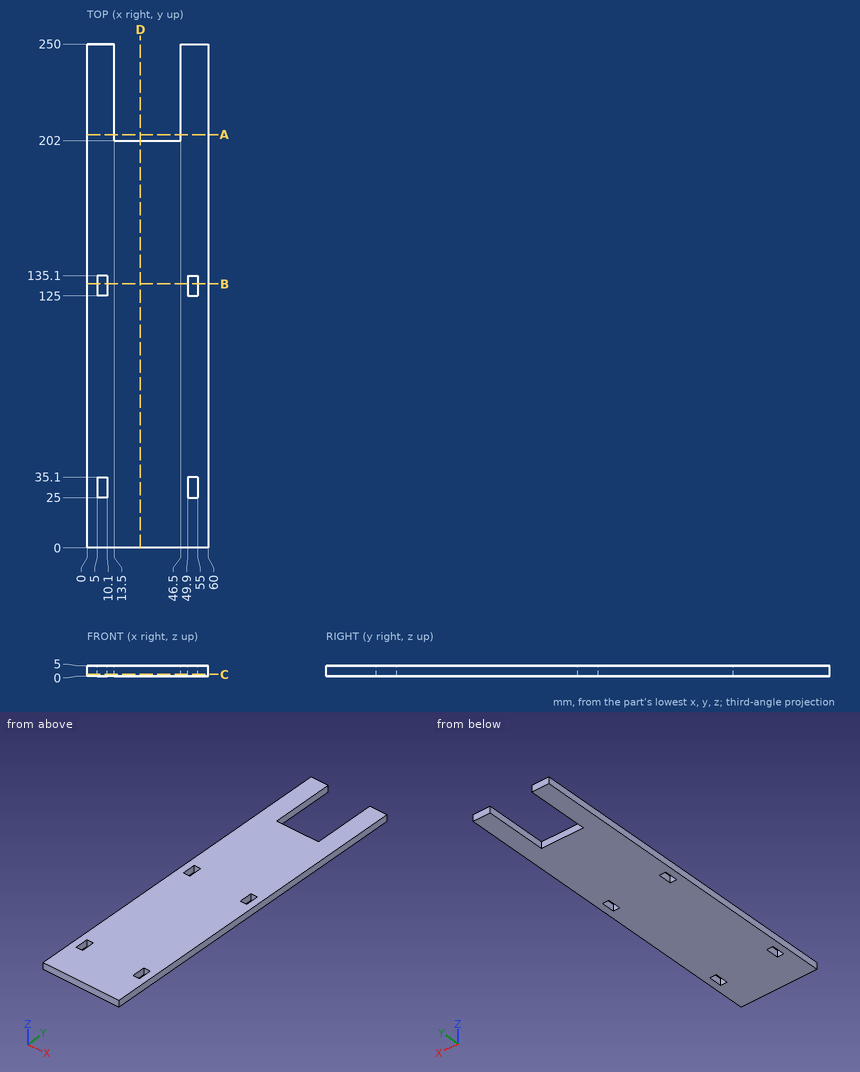
Input: dimensioned drawing with shaded views. Units: mm. Origin: part minimum x, y, z. Round coordinates to 2 decimals unless told otherwise and drop trailing zeros. Loops run counter-clockwise (first coordinate to the right, second up) from the corner with the lowest first, then second, coordinate; pieces in that order, holes last. Notation, with made-up numbers: (-2, -23) -> (29, -23) arc R36 cw to (29, 11) -> close; hole circle Ø9 at (50, 70.5). An arc over 180 degrees is marked (long way). Answer as a JSON object with one key per item and string values. Group by question number.
Q1. Section query C-C (z = 0.85). Output: boundary loops of the cut face in (x, y), plus the area to 3 significant figures.
Q2. Ray query, line 1 (X direction, y = 27, z = 1.2); line 2 (Y direction, x = 8.5, z = 3.55); line 3 (Y direction, x = 26.5, z = 0.3). Return the intervals inside material, ascending. Write a range as from..to.
Q3. Section query B-B (y = 131). Output: boundary loops of the cut face in (x, z), plus the area to 3 significant figures.
Q4. Section query A-A (y = 205). Output: boundary loops of the cut face in (x, z).
Q5. Contact query for a flat-ended pin moving along its axis: P1, Ø1.5, axis at x = 19.5, y = 111.5, coming from the -Z side. Output: stop coordinate, or through.
Q6. Section query D-D (x = 26.5). Output: boundary loops of the cut face in (y, z), plus the area to 3 significant figures.
Completed:
{
 "1": {"outline": "(0, 0) -> (60, 0) -> (60, 250) -> (46.5, 250) -> (46.5, 202) -> (13.5, 202) -> (13.5, 250) -> (0, 250) -> close; hole (5, 25) -> (10.1, 25) -> (10.1, 35.1) -> (5, 35.1) -> close; hole (5, 125) -> (10.1, 125) -> (10.1, 135.1) -> (5, 135.1) -> close; hole (49.9, 25) -> (55, 25) -> (55, 35.1) -> (49.9, 35.1) -> close; hole (49.9, 125) -> (55, 125) -> (55, 135.1) -> (49.9, 135.1) -> close", "area": "13,200 mm²"},
 "2": {"line 1": "0..5, 10.1..49.9, 55..60", "line 2": "0..25, 35.1..125, 135.1..250", "line 3": "0..202"},
 "3": {"outline": "(0, 0) -> (5, 0) -> (5, 5) -> (0, 5) -> close; (10.1, 0) -> (49.9, 0) -> (49.9, 5) -> (10.1, 5) -> close; (55, 0) -> (60, 0) -> (60, 5) -> (55, 5) -> close", "area": "249 mm²"},
 "4": {"outline": "(0, 0) -> (13.5, 0) -> (13.5, 5) -> (0, 5) -> close; (46.5, 0) -> (60, 0) -> (60, 5) -> (46.5, 5) -> close"},
 "5": {"P1": "z = 0"},
 "6": {"outline": "(0, 0) -> (202, 0) -> (202, 5) -> (0, 5) -> close", "area": "1,010 mm²"}
}
